The model under review builds one solid part; all positions refer to its coordinate system, in mm. Face numbers are marked on the shaded views. A direction names the side the tool comes from. Coordinates: 2 decimals unless noted, no trailing zeros. Write each loop counter-clockwise with the first axis right and the second up, starting at its lowest first coordinate (ties: lowest second). Pieces come first, ordered by that corner, then holes. Notation, with made-up numbers: M -34.5,40 L -11.5,40 A24 cw -11.5,79 Z; hole C -36,-12 d3. An arc over 180 degrees is marked long. Answer as a JSON object with one key per item and string values.
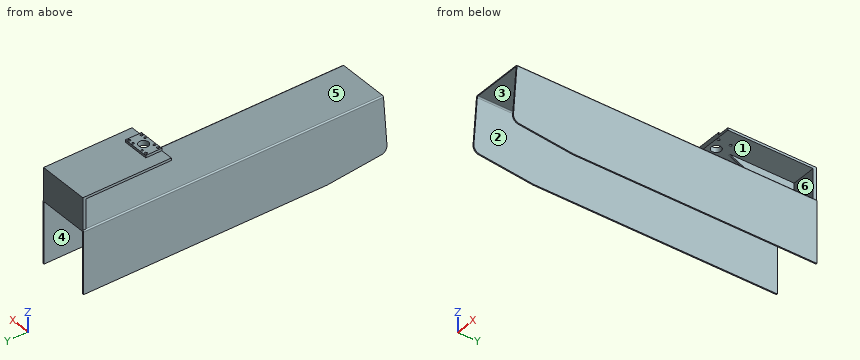
```python
from build123d import *

# Parameters (mm, degrees)
F1_DEPTH  = 600.075
F2_R      = 4.7625
F4_DEPTH  = 209.55
F6_DEPTH  = 209.55
F7_R      = 25.4
F9_DEPTH  = 101.6
F11_DEPTH = 3.175
F12_W     = 104.775
F12_H     = 63.5
F13_DEPTH = 9.525
F14_R     = 19.05
F14_R_2   = 4.7625
F15_DEPTH = 19.05
F16_R     = 3.96875
F17_DEPTH = 9.525


with BuildPart() as f1:
    # F0 (on Front) → F1 (new body, symmetric)
    with BuildSketch(Plane.XZ):
        Polygon((-104.775, -242.8875), (-100.0125, -242.8875), (-100.0125, 0), (100.0125, 0), (100.0125, -242.8875), (104.775, -242.8875), (104.775, 4.7625), (-104.775, 4.7625), align=None)
    extrude(amount=F1_DEPTH, both=True)

    # F2
    f2_edges = [f1.edges().sort_by_distance(p)[0] for p in [
        (-104.775, 0, 4.7625),
        (-100.0125, 0, 0),
        (104.775, 0, 4.7625),
        (100.0125, 0, 0),
    ]]
    fillet(f2_edges, radius=F2_R)

    # F3 (on face) → F4 (cut, through all)
    with BuildSketch(Plane(origin=(-104.775, 0, 0), x_dir=(0, -1, 0), z_dir=(-1, 0, 0))):
        Polygon((600.075, -242.8875), (600.075, -217.4875), (361.95, -242.8875), align=None)
    extrude(amount=-F4_DEPTH, mode=Mode.SUBTRACT)

    # F5 (on face) → F6 (cut, through all)
    with BuildSketch(Plane(origin=(-104.775, 0, 0), x_dir=(0, -1, 0), z_dir=(-1, 0, 0))):
        Polygon((584.2, 4.7625), (600.075, -217.4875), (600.075, 4.7625), align=None)
    extrude(amount=-F6_DEPTH, mode=Mode.SUBTRACT)

    # F7
    f7_edges = [f1.edges().sort_by_distance(p)[0] for p in [
        (-102.39375, -600.075, -217.4875),
        (102.39375, -600.075, -217.4875),
        (-102.39375, -361.95, -242.8875),
        (102.39375, -361.95, -242.8875),
    ]]
    fillet(f7_edges, radius=F7_R)

    # F8 (on Right) → F9 (join, symmetric)
    with BuildSketch(Plane.YZ):
        Polygon((587.375, 4.7625), (600.075, 4.7625), (600.075, 131.7625), (250.825, 131.7625), (250.825, 122.2375), (587.375, 122.2375), align=None)
    extrude(amount=F9_DEPTH, both=True)

    # F10 (on Right) → F11 (join, symmetric)
    with BuildSketch(Plane.YZ):
        Polygon((587.375, 4.7625), (587.375, 122.2375), (333.375, 122.2375), align=None)
    extrude(amount=F11_DEPTH, both=True)

    # F12 (on face) → F13 (join)
    with BuildSketch(Plane.XY.offset(131.7625)):
        with Locations((0, 282.575)):
            Rectangle(F12_W, F12_H)
    extrude(amount=F13_DEPTH)

    # F14 (on face) → F15 (cut, through all)
    with BuildSketch(Plane.XY.offset(141.2875)):
        with Locations((0, 282.575)):
            Circle(F14_R)
        with Locations((-42.8625, 306.3875)):
            Circle(F14_R_2)
        with Locations((-42.8625, 258.7625)):
            Circle(F14_R_2)
        with Locations((42.8625, 258.7625)):
            Circle(F14_R_2)
        with Locations((42.8625, 306.3875)):
            Circle(F14_R_2)
    extrude(amount=-F15_DEPTH, mode=Mode.SUBTRACT)

    # F16 (on face) → F17 (cut, through all)
    with BuildSketch(Plane.XY.offset(141.2875)):
        with Locations((-23.8125, 306.3875)):
            Circle(F16_R)
        with Locations((23.8125, 306.3875)):
            Circle(F16_R)
        with Locations((23.8125, 258.7625)):
            Circle(F16_R)
        with Locations((-23.8125, 258.7625)):
            Circle(F16_R)
    extrude(amount=-F17_DEPTH, mode=Mode.SUBTRACT)


solid = f1.part
```
(1) Add section B-B on z = -166. Give the boundary of the cut face in (x, y) (1 decimal).
Results list:
{"outline": "M -104.8,-596.4 L -100,-596.4 L -100,600.1 L -104.8,600.1 Z; M 100,-596.4 L 104.8,-596.4 L 104.8,600.1 L 100,600.1 Z"}
(2) Add section C-C on x = -74.5. Give the boundary of the cut face in (y, z) (1 decimal), and give its area (3 significant figures).
Results list:
{"outline": "M -584.5,0 L 600.1,0 L 600.1,131.8 L 250.8,131.8 L 250.8,122.2 L 587.4,122.2 L 587.4,4.8 L -584.2,4.8 Z", "area": "10,500 mm²"}
(3) For the marked faces 4, 5 and 6, list the 3-axis set-ups (+Z, -Z, +X, -X, +Y, -Y) from which the entire face can be reached by the end or side of a thin tool; tool diameter is ignored.
Results list:
{"face 4": "-Z, +Y, -Y", "face 5": "+X, -X, -Y", "face 6": "+X, -Y"}
(4) For pin 1 Ø8.5 at (x, y) = (-42.86, 258.76) entering from -Z; pin 2 Ø1 at (x, y) = (-24, 232.5) entering from +Z; pin 3 Ø10 at (x, y) = (0, 373.5) entering from +Z, all flat-tipped, find the tip position at first contact; note any pin that passes through.
Results list:
{"pin 1": "z = 0", "pin 2": "z = 4.76", "pin 3": "z = 131.76"}
(5) Draft analysis for pull direction Z (two halves, no side actions). For the marked faces 1, 2 and 3, state which applies: released by +Z, released by -Z, zero draft, split by the parting line, or undercut.
Results list:
{"face 1": "undercut", "face 2": "zero draft", "face 3": "released by -Z"}
(6) Add section D-D on z = 57.5. Give the boundary of the cut face in (x, y) (3 decimals).
Results list:
{"outline": "M -101.6,587.375 L -3.175,587.375 L -3.175,473.348 L 3.175,473.348 L 3.175,587.375 L 101.6,587.375 L 101.6,600.075 L -101.6,600.075 Z"}
(7) Wall thickness on line 1 along X through (y, z) = (-175.5, -97.5) (1 decimal); line 2 along Z through (x, y) = (-71, 497); line 3 along Y through (x, z) = (8.5, 2) (3 decimals): over which ranges is each line inside the solid? List them lowest first. Write a range as from..to.
Results list:
{"line 1": "-104.8..-100, 100..104.8", "line 2": "0..4.76, 122.24..131.76", "line 3": "-584.397..600.075"}
